Input: part model. Units: mm. Frame: model coordinates. Face numbers are marked on the shaded views. A direction names the side the tool comes from. Round coordinates to 2 decimals unless told otherwise and drop trailing zeros. Write each loop counter-clockwise with the first axis right and the second up, starting at its lowest first coordinate (ties: lowest second). Pieces come first, ordered by that corner, then holes. Notation, with made-up numbers: (40.5, -26) -> (64.5, -26) arc R21 cw to (64.5, -3) -> close; hole circle Ø7 at (32.25, -15.75). An arc over 180 degrees is marked (long way). Use CSV: the item, a comma, the result in double quotes.
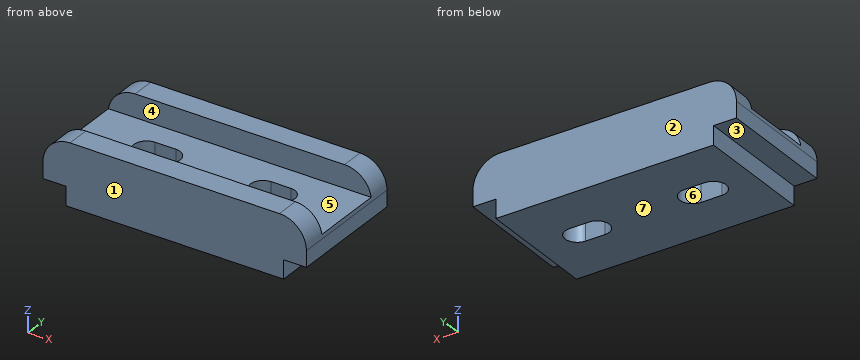
```python
from build123d import *

# Parameters (mm, degrees)
F1_DEPTH = 58
F4_DEPTH = 29.741798
F6_DEPTH = 11


with BuildPart() as f1:
    # F0 (on Front) → F1 (new body)
    with BuildSketch(Plane.XZ):
        with BuildLine():
            Line((-52.5, 9), (-52.5, 0))
            Line((-52.5, 0), (52.5, 0))
            Line((52.5, 0), (52.5, 9))
            Line((52.5, 9), (63.5, 9))
            Line((63.5, 9), (63.5, 16.740798))
            ThreePointArc((63.5, 16.740798), (59.692388, 25.933186), (50.5, 29.740798))
            Line((50.5, 29.740798), (-50.5, 29.740798))
            ThreePointArc((-50.5, 29.740798), (-59.692388, 25.933186), (-63.5, 16.740798))
            Line((-63.5, 16.740798), (-63.5, 9))
            Line((-63.5, 9), (-52.5, 9))
        make_face()
    extrude(amount=F1_DEPTH)

    # F3 (on face) → F4 (cut, through all)
    with BuildSketch(Plane.XY.offset(29.740798)):
        with BuildLine():
            Line((-22.874139, -22.915082), (-32.964889, -22.915082))
            ThreePointArc((-32.964889, -22.915082), (-39.049807, -29), (-32.964889, -35.084918))
            Line((-32.964889, -35.084918), (-22.874139, -35.084918))
            ThreePointArc((-22.874139, -35.084918), (-16.789221, -29), (-22.874139, -22.915082))
        make_face()
        with BuildLine():
            Line((32.622553, -23.102847), (23.132133, -23.102847))
            ThreePointArc((23.132133, -23.102847), (17.234981, -29), (23.132133, -34.897153))
            Line((23.132133, -34.897153), (32.622553, -34.897153))
            ThreePointArc((32.622553, -34.897153), (38.519706, -29), (32.622553, -23.102847))
        make_face()
    extrude(amount=-F4_DEPTH, mode=Mode.SUBTRACT)

    # F5 (on face) → F6 (cut)
    with BuildSketch(Plane.XY.offset(29.740798)):
        Polygon((63.615084, -11.138136), (-63.967951, -11.138136), (-63.786983, -46.608031), (63.615084, -46.608031), align=None)
    extrude(amount=-F6_DEPTH, mode=Mode.SUBTRACT)


solid = f1.part
```
Item 1: Section query D-D on y = -44. Return the cut outline in (x, z).
Worked answers:
outline,"(-63.5, 9) -> (-52.5, 9) -> (-52.5, 0) -> (52.5, 0) -> (52.5, 9) -> (63.5, 9) -> (63.5, 16.74) arc R13 ccw to (63.35, 18.74) -> (-63.35, 18.74) arc R13 ccw to (-63.5, 16.74) -> close"
Item 2: Line query: line 1 (Y direction, x = 15.5, z = 21.75); line 2 (X direction, y = -30.5, z = 13.5); line 3 (X direction, y = -30, z = 11). Output: solid intervals per line, ascending.
Worked answers:
line 1,"y = -58 to -46.61, -11.14 to 0"
line 2,"x = -63.5 to -38.86, -16.98 to 17.43, 38.33 to 63.5"
line 3,"x = -63.5 to -38.97, -16.87 to 17.32, 38.43 to 63.5"
Item 3: Section query A-A on y = -29. Return the cut outline in (x, z).
Worked answers:
outline,"(-63.5, 9) -> (-52.5, 9) -> (-52.5, 0) -> (-39.05, 0) -> (-39.05, 18.74) -> (-63.35, 18.74) arc R13 ccw to (-63.5, 16.74) -> close; (-16.79, 0) -> (17.23, 0) -> (17.23, 18.74) -> (-16.79, 18.74) -> close; (38.52, 0) -> (52.5, 0) -> (52.5, 9) -> (63.5, 9) -> (63.5, 16.74) arc R13 ccw to (63.35, 18.74) -> (38.52, 18.74) -> close"
Item 4: Section query B-B on x = 29.5. Return the cut outline in (y, z), plus the area to 3 significant figures.
Worked answers:
outline,"(-58, 0) -> (-34.9, 0) -> (-34.9, 18.74) -> (-46.61, 18.74) -> (-46.61, 29.74) -> (-58, 29.74) -> close; (-23.1, 0) -> (0, 0) -> (0, 29.74) -> (-11.14, 29.74) -> (-11.14, 18.74) -> (-23.1, 18.74) -> close"
area,"1,110 mm²"
Item 5: Set-up query: the marked faces 5, 6 and 7. Return all of +Z, -Z, +X, -X, +Y, -Y with unobstructed straight access to the full face (end or side cutting, diameter ignored); none if empty.
Worked answers:
face 5,"+Z, +X, -X"
face 6,"+Z, -Z"
face 7,"-Z, +X, -X, +Y, -Y"
Item 6: Pull-direction query (Y, two-part tool) for the marked faces 1, 2, 3 and 4; classes: +Y half, -Y half, draft (parallel to the pull), parting line (faces both ways), or undercut.
Worked answers:
face 1,"-Y half"
face 2,"+Y half"
face 3,"draft"
face 4,"undercut"
Item 7: Section query C-C on z = 14. Return the cut outline in (x, y).
Worked answers:
outline,"(-63.5, -58) -> (63.5, -58) -> (63.5, 0) -> (-63.5, 0) -> close; hole (-32.96, -35.08) -> (-22.87, -35.08) arc R6.08 ccw to (-22.87, -22.92) -> (-32.96, -22.92) arc R6.08 ccw to start; hole (23.13, -34.9) -> (32.62, -34.9) arc R5.9 ccw to (32.62, -23.1) -> (23.13, -23.1) arc R5.9 ccw to start"
Item 8: First-contact query: pin 1 Ø3.5 at (x, y) = (-59, -35) entering from -Z; pin 2 Ø5.5 at (x, z) = (6, 24.5) entering from +Y; pin 3 Ø2.5 at (y, z) = (-35.5, 6) entering from +X; pin 4 Ø7 at (y, z) = (-43, 3.5) entering from -X. Flat tips, straight axial feed; report the tip coordinate or a pass-through.
Worked answers:
pin 1,"stops at z = 9"
pin 2,"stops at y = 0"
pin 3,"stops at x = 52.5"
pin 4,"stops at x = -52.5"
